from build123d import *

# Parameters (mm, degrees)
SKICA2_R                                         = 11.5
P_IDAT_VYSUNUT_M1_DEPTH                          = 15
SKICA5_W                                         = 55
SKICA5_H                                         = 5
P_IDAT_VYSUNUT_M4_DEPTH                          = 11.5
ZKOSEN_1_SIZE                                    = 1
SKICA6_W                                         = 43.3
SKICA6_H                                         = 43.3
ODEBRAT_VYSUNUT_M1_DEPTH                         = 4.5
V_LCOV_ZAHLOUBEN_PRO_M3_ROUBY_S_VNIT_D           = 3.5
V_LCOV_ZAHLOUBEN_PRO_M3_ROUBY_S_VNIT_CBORE_D     = 6.5
V_LCOV_ZAHLOUBEN_PRO_M3_ROUBY_S_VNIT_CBORE_DEPTH = 3.7
SKICA10_W                                        = 55
SKICA10_H                                        = 5
P_IDAT_VYSUNUT_M5_DEPTH                          = 10
ZAOBLIT1_R                                       = 2
ZAOBLIT2_R                                       = 3


with BuildPart() as part:
    # Skica2 → Přidat vysunutím1 (new body)
    with BuildSketch(Plane.XY):
        with BuildLine():
            Line((-27.5, 24.5), (-27.5, -72.5))
            Line((-27.5, -72.5), (27.5, -72.5))
            Line((27.5, -72.5), (27.5, 24.5))
            ThreePointArc((27.5, 24.5), (26.621320344, 26.621320344), (24.5, 27.5))
            Line((24.5, 27.5), (-24.5, 27.5))
            ThreePointArc((-24.5, 27.5), (-26.621320344, 26.621320344), (-27.5, 24.5))
        make_face()
        Circle(SKICA2_R, mode=Mode.SUBTRACT)
    extrude(amount=-P_IDAT_VYSUNUT_M1_DEPTH)

    # Skica5 → Přidat vysunutím4 (add)
    with BuildSketch(Plane.XZ.offset(72.5)):
        with Locations((0, -2.5)):
            Rectangle(SKICA5_W, SKICA5_H)
    extrude(amount=P_IDAT_VYSUNUT_M4_DEPTH)

    # Zkosení1
    zkosen_1_edges = [part.edges().sort_by_distance(p)[0] for p in [
        (-27.5, -84, -2.5),
        (27.5, -84, -2.5),
    ]]
    chamfer(zkosen_1_edges, length=ZKOSEN_1_SIZE)

    # Skica6 → Odebrat vysunutím1 (cut)
    with BuildSketch(Plane(origin=(0, 0, -15), x_dir=(-1, 0, 0), z_dir=(0, 0, -1))):
        Rectangle(SKICA6_W, SKICA6_H)
    extrude(amount=-ODEBRAT_VYSUNUT_M1_DEPTH, mode=Mode.SUBTRACT)

    # Válcové zahloubení pro M3 šrouby s vnitřním šestihranem1 (through all)
    with Locations(Plane.XY):
        with Locations((15.5, 15.5), (-15.5, -15.5), (-15.5, 15.5), (15.5, -15.5)):
            CounterBoreHole(V_LCOV_ZAHLOUBEN_PRO_M3_ROUBY_S_VNIT_D / 2, V_LCOV_ZAHLOUBEN_PRO_M3_ROUBY_S_VNIT_CBORE_D / 2, V_LCOV_ZAHLOUBEN_PRO_M3_ROUBY_S_VNIT_CBORE_DEPTH)

    # Skica10 → Přidat vysunutím5 (add)
    with BuildSketch(Plane(origin=(0, 0, -15), x_dir=(-1, 0, 0), z_dir=(0, 0, -1))):
        with Locations((0, -70)):
            Rectangle(SKICA10_W, SKICA10_H)
    extrude(amount=P_IDAT_VYSUNUT_M5_DEPTH)

    # Zaoblit1
    zaoblit1_edges = [part.edges().sort_by_distance(p)[0] for p in [
        (27.5, -70, -25),
        (-27.5, -70, -25),
    ]]
    fillet(zaoblit1_edges, radius=ZAOBLIT1_R)

    # Zaoblit2
    zaoblit2_edges = [part.edges().sort_by_distance(p)[0] for p in [
        (0, -67.5, -15),
    ]]
    fillet(zaoblit2_edges, radius=ZAOBLIT2_R)


solid = part.part
Geometry check sheet. Reference: the model listing, model coordinates, mm. A direction names the side the tool comes from. Round coordinates to 2 decimals unless told otherwise and drop trailing zeros. Write each loop counter-clockwise with the first axis right and the second up, starting at its lowest first coordinate (ties: lowest second). Pieces come first, ordered by that corner, then holes.
Item 1: Section check C-C (x = 0). Record the boundary of the cut face in (y, z), plus the area to 3 significant figures.
Determined:
outline: (-84, -5) - (-72.5, -5) - (-72.5, -25) - (-67.5, -25) - (-67.5, -18) arc R3 cw to (-64.5, -15) - (-21.65, -15) - (-21.65, -10.5) - (-11.5, -10.5) - (-11.5, 0) - (-84, 0) - close; (11.5, -10.5) - (21.65, -10.5) - (21.65, -15) - (27.5, -15) - (27.5, 0) - (11.5, 0) - close
area: 1,170 mm2
Item 2: Section check B-B (x = -15.5). Give the number of separate pieces and of enclosed holes in the cut face, plus the area to 3 significant figures.
Determined:
separate pieces: 3
enclosed holes: 0
area: 1,320 mm2
Item 3: Mould release check, pull along Y, two halves, no side actions. Record for faces 1 (the face through (-9, -9, -10.5)), 2 (the face through (0, -67.5, -21)), 3 (the face through (0, -70, -25)): +Y half, -Y half, draft (parallel to the pull), parting line (faces both ways), or undercut.
Determined:
face 1: undercut
face 2: +Y half
face 3: draft
Item 4: Section check A-A (y = 0). Record the boundary of the cut face in (x, z), plus the area to 3 significant figures.
Determined:
outline: (-27.5, -15) - (-21.65, -15) - (-21.65, -10.5) - (-11.5, -10.5) - (-11.5, 0) - (-27.5, 0) - close; (11.5, -10.5) - (21.65, -10.5) - (21.65, -15) - (27.5, -15) - (27.5, 0) - (11.5, 0) - close
area: 389 mm2
Item 5: Section check D-D (y = 15.5). Record the boundary of the cut face in (x, z).
Determined:
outline: (-27.5, -15) - (-21.65, -15) - (-21.65, -10.5) - (-17.25, -10.5) - (-17.25, -3.7) - (-18.75, -3.7) - (-18.75, 0) - (-27.5, 0) - close; (-13.75, -10.5) - (13.75, -10.5) - (13.75, -3.7) - (12.25, -3.7) - (12.25, 0) - (-12.25, 0) - (-12.25, -3.7) - (-13.75, -3.7) - close; (17.25, -10.5) - (21.65, -10.5) - (21.65, -15) - (27.5, -15) - (27.5, 0) - (18.75, 0) - (18.75, -3.7) - (17.25, -3.7) - close
Item 6: Go/stop test with flat-tipped pins: pin 1 Ø2 at (x, z) = (-2.5, -13) entering from -Y; pin 2 Ø3 at (x, y) = (15.5, -15.5) entering from -Z; pin 3 Ø5 at (x, z) = (9, -22) entering from +Y; pin 4 Ø2 at (x, y) = (14.5, -15) entering from +Z. Record where each tip stops, or that it passes through.
Determined:
pin 1: stops at y = -72.5
pin 2: passes through
pin 3: stops at y = -67.5
pin 4: stops at z = -3.7
Item 7: Material ranges on line 1 along Y through (x, z) = (15.5, -9); line 2 along Y through (x, z) = (-15.5, -2.5); line 3 along Y through (x, z) = (14, -11.75), recorded low to high.
Determined:
line 1: y = -72.5 to -17.25, -13.75 to 13.75, 17.25 to 27.5
line 2: y = -84 to -18.75, -12.25 to 12.25, 18.75 to 27.5
line 3: y = -72.5 to -21.65, 21.65 to 27.5
Item 8: Access from +Z, -Z, +X, -X, +Y, -Y to the whole of each face (thin tool, end or side, straight path). Record for faces 4 (the face through (0, -27, 0)), 5 (the face through (-15.923, -12.278, -1.824)), 6 (the face through (0, -78, -5)), 7 (the face through (26.93, -69.96, -24.4)), 8 (the face through (21.65, 0, -13)).
Determined:
face 4: +Z, +X, -X, +Y, -Y
face 5: +Z
face 6: -Z, +X, -X, -Y
face 7: -Z, +X, +Y, -Y
face 8: -Z
